Verification items for the finished model (mm, model axes). Give positions to 0.01 mm unless a question says otherwise; leave off trailing zeros. Order: outer loops, then holes, each group sorted by start corner. A loop starts at its lowest first (then second) coordinate and runs counter-clockwise, first axis right, second up.
from build123d import *

# Parameters (mm, degrees)
SKETCH1_W                = 47.6
SKETCH1_H                = 5.8
BOSS_EXTRUDE1_DEPTH      = 2
M3_CLEARANCE_HOLE1_D     = 3.2
M3_CLEARANCE_HOLE1_DEPTH = 3


with BuildPart() as part:
    # Sketch1 → Boss-Extrude1 (new body)
    with BuildSketch(Plane(origin=(0, 0, 0), x_dir=(1, 0, 0), z_dir=(0, 1, 0))):
        with Locations((24, 2.9)):
            Rectangle(SKETCH1_W, SKETCH1_H)
        with Locations((24, 8.7)):
            Rectangle(SKETCH1_W, SKETCH1_H)
    extrude(amount=BOSS_EXTRUDE1_DEPTH)

    # M3 Clearance Hole1
    with Locations(Plane(origin=(0, 2, 0), x_dir=(1, 0, 0), z_dir=(0, 1, 0))):
        with Locations((42, 5.8), (30, 5.8), (18, 5.8), (6, 5.8)):
            Hole(M3_CLEARANCE_HOLE1_D / 2, depth=M3_CLEARANCE_HOLE1_DEPTH)


solid = part.part
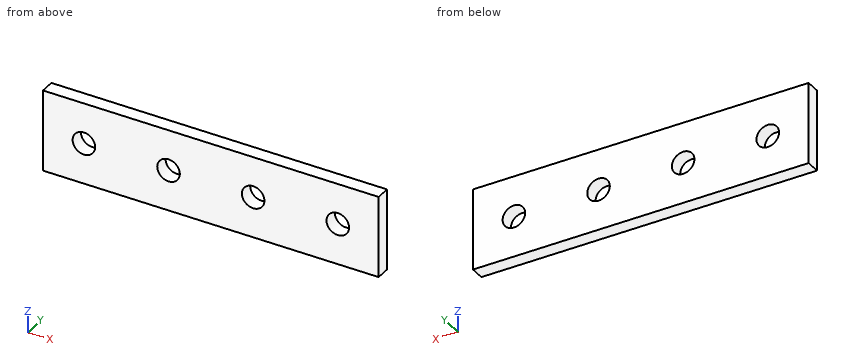
(1) Scan lines: line 1 (X direction, y = 0.95, z = -5.8); line 2 (Z direction, x = 30, y = 1.55); line 3 (X direction, y = 1.55, z = -7.25). Record each from-to range of solid material in increasing order.
Solved:
line 1: x = 0.2 to 4.4, 7.6 to 16.4, 19.6 to 28.4, 31.6 to 40.4, 43.6 to 47.8
line 2: z = -11.6 to -7.4, -4.2 to 0
line 3: x = 0.2 to 5.32, 6.68 to 17.32, 18.68 to 29.32, 30.68 to 41.32, 42.68 to 47.8
(2) Go/stop test with a flat-tipped pin: pin 1 (1 mm diameter, centred on x = 20, y = 1, fed in from +Z). Record where the tip stops, or that it passes through.
Solved:
pin 1: stops at z = 0
(3) Section check C-C, the plane z = -7. Enter the section's corners in (x, y), then the cut area to 3 significant figures.
Solved:
outline: (0.2, 0) - (4.94, 0) - (4.94, 2) - (0.2, 2) - close; (7.06, 0) - (16.94, 0) - (16.94, 2) - (7.06, 2) - close; (19.06, 0) - (28.94, 0) - (28.94, 2) - (19.06, 2) - close; (31.06, 0) - (40.94, 0) - (40.94, 2) - (31.06, 2) - close; (43.06, 0) - (47.8, 0) - (47.8, 2) - (43.06, 2) - close
area: 78.3 mm2
(4) Section check A-A, the plane x = 6. Enter the section's corners in (y, z).
Solved:
outline: (0, -11.6) - (2, -11.6) - (2, -7.4) - (0, -7.4) - close; (0, -4.2) - (2, -4.2) - (2, 0) - (0, 0) - close
(5) Section check B-B, the plane y = 0.65. Enter the section's corners in (x, z).
Solved:
outline: (0.2, -11.6) - (47.8, -11.6) - (47.8, 0) - (0.2, 0) - close; hole circle Ø3.2 at (6, -5.8); hole circle Ø3.2 at (18, -5.8); hole circle Ø3.2 at (30, -5.8); hole circle Ø3.2 at (42, -5.8)
